from build123d import *

# Parameters (mm, degrees)
SKETCH1_R           = 15
SKETCH1_R_2         = 6
BOSS_EXTRUDE1_DEPTH = 60
SKETCH2_R           = 15
SKETCH5_R           = 20
BOSS_EXTRUDE2_DEPTH = 100


with BuildPart() as part:
    # Sketch1 → Boss-Extrude1 (new, symmetric)
    with BuildSketch(Plane.XY):
        Circle(SKETCH1_R)
        Circle(SKETCH1_R_2, mode=Mode.SUBTRACT)
    extrude(amount=BOSS_EXTRUDE1_DEPTH, both=True)

    # Sweep1: sweep along a path in Sketch3
    with BuildLine(Plane.XY) as sweep1_path:
        Line((0, 0), (500, 0))
        Line((500, 0), (969.846310393, 171.010071663))
    # Sketch2 → Sweep1 (sweep)
    with BuildSketch(Plane(origin=(0, 0, 0), x_dir=(0, 0, -1), z_dir=(1, 0, 0))):
        Circle(SKETCH2_R)
    sweep(path=sweep1_path.line, transition=Transition.RIGHT)

    # Sketch5 → Boss-Extrude2 (add, symmetric)
    with BuildSketch(Plane.XY):
        with Locations((969.846310393, 171.010071663)):
            Circle(SKETCH5_R)
    extrude(amount=BOSS_EXTRUDE2_DEPTH, both=True)


solid = part.part
Design review of the part built by this model. Coordinates are the model's own, in mm. A direction names the side the tool comes from. Give positions to 0.01 mm unless a question says otherwise; leave off trailing zeros. Write each loop counter-clockwise with the first axis right and the second up, starting at its lowest first coordinate (ties: lowest second). Pieces come first, ordered by that corner, then holes. Notation, with made-up numbers: M -23.75,69.5 L -7.75,69.5 A12 cw -7.75,76.5 Z; hole C 82,44 d10. An arc over 180 degrees is marked long. Answer as a JSON object with one key per item and string values. Group by question number.
1) We need section A-A (z = 0). Give the boundary of the cut face in (x, y).
2) Tool access review of faces 1 (the face through (970, 171, 100)), 2 (the face through (255, -9, 12)): name each direction out of +Z, -Z, +X, -X, +Y, -Y from which nothing blocks a thin tool from reaching the whole face with its end or side.
3) We need section C-C (x = 98). Give the boundary of the cut face in (y, z).
4) For line 1 along Y through (x, z) = (0, 29.5); line 2 along Y through (x, z) = (222, 10); line 3 along X through (y, z) = (-4.5, -31), list the stretches that pass through material, from the lowest coordinate up.
5) Clearance check with flat-ended pins moving along their axes: pin 1 Ø11 at (x, y) = (0, 0) entering from +Z; pin 2 Ø8 at (y, z) = (99, -22.5) entering from -X; pin 3 Ø9 at (x, y) = (-6.5, -7) entering from +Z. State where each tip first meets the part, or that it passes through.
6) We need section D-D (z = -72.5). Give the boundary of the cut face in (x, y), and give its area (3 significant figures).
7) We need section B-B (z = 40). Give the boundary of the cut face in (x, y), and give its area (3 significant figures).
Answer key:
{
 "1": {"outline": "M 0,-15 L 502.64,-15 L 962.55,152.39 A20 ccw long 952.29,180.58 L 497.36,15 L 0,15 A15 ccw Z; hole M 0,-6 L 0,6 A6 ccw Z"},
 "2": {"face 1": "+Z, +X, -X, +Y, -Y", "face 2": "none"},
 "3": {"outline": "C 0,0 d30"},
 "4": {"line 1": "y = -15 to -6, 6 to 15", "line 2": "y = -11.18 to 11.18", "line 3": "x = -14.31 to -3.97, 3.97 to 14.31"},
 "5": {"pin 1": "stops at z = 15", "pin 2": "passes through", "pin 3": "stops at z = 60"},
 "6": {"outline": "C 969.85,171.01 d40", "area": "1,260 mm²"},
 "7": {"outline": "C 0,0 d30; C 969.85,171.01 d40; hole C 0,0 d12", "area": "1,850 mm²"}
}
